```python
from build123d import *

# Parameters (mm, degrees)
F1_DEPTH = 3
F0_W     = 3
F0_H     = 0.2339549768
F2_DEPTH = 6
F3_W     = 3
F3_H     = 1
F4_DEPTH = 3
F5_R     = 0.99999
F6_SIZE  = 2


# Not quite as in the source:
# - a fillet or chamfer is up to 0.001 mm smaller than in the source, because OpenCascade refuses the exact size
# - a feature names something its author has since deleted; it is built from what else it names


with BuildPart() as f1:
    # F0 (on Top) → F1 (new body)
    with BuildSketch(Plane.XY):
        with BuildLine():
            Line((-2.5, 70), (2.5, 70))
            ThreePointArc((2.5, 70), (0, 70.139320225), (-2.5, 70))
        make_face()
        with BuildLine():
            ThreePointArc((22.5, 47.639320225), (16.7705098312, 62.639320225), (2.5, 70))
            Line((2.5, 70), (2.5, 64.9598283007))
            ThreePointArc((2.5, 64.9598283007), (13.2287565553, 59.0957594624), (17.5, 47.639320225))
            ThreePointArc((17.5, 47.639320225), (13.2287565553, 36.1828809876), (2.5, 30.3188121493))
            Line((2.5, 30.3188121493), (2.5, 25.27864045))
            ThreePointArc((2.5, 25.27864045), (16.7705098312, 32.639320225), (22.5, 47.639320225))
        make_face()
        with BuildLine():
            Line((-2.5, 64.9598283007), (-2.5, 70))
            ThreePointArc((-2.5, 70), (-22.5, 47.639320225), (-2.5, 25.27864045))
            Line((-2.5, 25.27864045), (-2.5, 30.3188121493))
            ThreePointArc((-2.5, 30.3188121493), (-17.5, 47.639320225), (-2.5, 64.9598283007))
        make_face()
        with BuildLine():
            Line((2.5, 64.9598283007), (2.5, 70))
            Line((2.5, 70), (-2.5, 70))
            Line((-2.5, 70), (-2.5, 64.9598283007))
            ThreePointArc((-2.5, 64.9598283007), (0, 65.139320225), (2.5, 64.9598283007))
        make_face()
        with BuildLine():
            Line((-2.5, 30.3188121493), (-2.5, 25.27864045))
            ThreePointArc((-2.5, 25.27864045), (0, 25.139320225), (2.5, 25.27864045))
            Line((2.5, 25.27864045), (2.5, 30.3188121493))
            ThreePointArc((2.5, 30.3188121493), (0, 30.139320225), (-2.5, 30.3188121493))
        make_face()
        with BuildLine():
            Line((-1.5, -65.5), (-2.5, -65.5))
            Line((-2.5, -65.5), (-2.5, -67.5))
            ThreePointArc((-2.5, -67.5), (-1.767766953, -69.267766953), (0, -70))
            ThreePointArc((0, -70), (1.767766953, -69.267766953), (2.5, -67.5))
            Line((2.5, -67.5), (2.5, -65.5))
            Line((2.5, -65.5), (1.5, -65.5))
            Line((1.5, -65.5), (1.5, -65.7339549768))
            Line((1.5, -65.7339549768), (-1.5, -65.7339549768))
            Line((-1.5, -65.7339549768), (-1.5, -65.5))
        make_face()
        with BuildLine():
            ThreePointArc((2.5, 25.27864045), (0, 25.139320225), (-2.5, 25.27864045))
            Line((-2.5, 25.27864045), (-2.5, -65.5))
            Line((-2.5, -65.5), (-1.5, -65.5))
            Line((-1.5, -65.5), (-1.5, -65.2660450232))
            Line((-1.5, -65.2660450232), (1.5, -65.2660450232))
            Line((1.5, -65.2660450232), (1.5, -65.5))
            Line((1.5, -65.5), (2.5, -65.5))
            Line((2.5, -65.5), (2.5, 25.27864045))
        make_face()
    extrude(amount=F1_DEPTH)

    # F0 (on Top) → F2 (join)
    with BuildSketch(Plane.XY):
        with Locations((0, -65.3830225116)):
            Rectangle(F0_W, F0_H)
        with Locations((0, -65.6169774884)):
            Rectangle(F0_W, F0_H)
    extrude(amount=F2_DEPTH)

    # F3 (on face) → F4 (join)
    with BuildSketch(Plane(origin=(0, -65.2660450232, 0), x_dir=(-1, 0, 0), z_dir=(0, 1, 0))):
        with Locations((0, 5.5)):
            Rectangle(F3_W, F3_H)
    extrude(amount=F4_DEPTH)

    # F5 (radius 1 in the source; OpenCascade refuses exactly that, so slightly less here)
    f5_edges = [f1.edges().sort_by_distance(p)[0] for p in [
        (0, 70.13932, 3),
        (0, 70.13932, 0),
        (2.5, -21.11068, 0),
        (2.5, -21.11068, 3),
        (-2.5, -21.11068, 3),
        (-2.5, -21.11068, 0),
    ]]
    fillet(f5_edges, radius=F5_R)

    # F6
    f6_edges = [f1.edges().sort_by_distance(p)[0] for p in [
        (-2.5, 64.959828, 3),
    ]]
    chamfer(f6_edges, length=F6_SIZE)


solid = f1.part
```
Geometry: final body of the model. Coordinates: model frame, mm. A direction names the side the tool comes from. Round coordinates to 2 decimals unless told otherwise and drop trailing zeros. Write each loop counter-clockwise with the first axis right and the second up, starting at its lowest first coordinate (ties: lowest second). Pieces come first, ordered by that corner, then holes.
Item 1: Section query A-A (y = 13). Return loops of the section in (x, z), plus the area to 3 significant figures.
Item 2: Material intervals for L1, parallel to Z at x = 0.5, y = -30.5; L2, parallel to Y at x = -2, z = 0.5; L3, parallel to Y at x = 5, z = 2, sorted ascending.
Item 3: Mould query, pull axis Z, two halves, no side actions, for faces 4 (the face through (0, -64, 5)), 5 (the face through (0, 21, 0)), 6 (the face through (0, -64, 6)). Classes: +Z half, -Z half, draft (parallel to the pull), parting line (faces both ways), or undercut.
Item 4: Set-up query: faces 1 (the face through (-1.5, -64.41, 5.15)), 2 (the face through (1.5, -64.41, 5.15)), 3 (the face through (0, -65.734, 4)). Return all of +Z, -Z, +X, -X, +Y, -Y with unobstructed straight access to the full face (end or side cutting, diameter ignored); none if empty.
Item 5: Pin query (flat end, axial travel): P1, Ø0.6, axis at x = 0.5, z = 4, coming from the +Y side; P2, Ø3.5, axis at x = -0.5, z = 4, coming from the -Y side; P3, Ø2.5, axis at y = -65, z = 4, coming from the +X side; P4, Ø4, axis at x = 13.5, y = 54.5, coming from the -Z side. Return the tip coordinate at first contact, or that it passes through.
Completed:
1. outline: (-2.5, 1) arc R1 ccw to (-1.5, 0) - (1.5, 0) arc R1 ccw to (2.5, 1) - (2.5, 2) arc R1 ccw to (1.5, 3) - (-1.5, 3) arc R1 ccw to (-2.5, 2) - close
1. area: 14.1 mm2
2. L1: z = 0 to 3
2. L2: y = -68.76 to 30.25, 65.02 to 69.92
2. L3: y = 25.7 to 29.83, 65.45 to 69.58
3. face 4: undercut
3. face 5: -Z half
3. face 6: +Z half
4. face 1: +Z, -X, +Y, -Y
4. face 2: +Z, +X, +Y, -Y
4. face 3: +Z, +X, -X, -Y
5. P1: stops at y = -65.27
5. P2: stops at y = -69.95
5. P3: stops at x = 2.16
5. P4: passes through
